The listing builds one solid part. Answer for the finished solid, in the listing's coordinates (mm). Coordinates: 2 decimals unless noted, no trailing zeros. Order: outer loops, then holes, each group sorted by start corner. A loop starts at its lowest first (then second) coordinate and runs counter-clockwise, first axis right, second up. Notation, with made-up numbers: (81.25, 82) - (109.25, 82) arc R27 ccw to (109.25, 100) - close; hole circle Ø6 at (10.25, 74.5). An arc over 180 degrees is marked (long way). Use one line per item in the form item = value. Start each with the question number.
Item 1: Section A-A, the plane z = 0 is taken. Write down the section's boundary in (x, y).
Item 2: The mould has two halves that part along Z. Classify faces 1 (the flat face through (0, 2, 25)), 2 (the flat face through (0, 0, 0)), 3 (the cylindrical face through (3.583, 2.169, -0.759)), 4 (the cylindrical face through (-10.417, 2.169, -0.759)): released by +Z, released by -Z, zero draft, split by the parting line, or undercut.
Item 3: Consider line 1 along X through (y, z) = (2.3, 0); line 2 along X through (y, z) = (3.45, -3); line 3 along Z through (x, y) = (8, 3.4). Determine where each line is inside the solid, lowest interval first. Write a range as [from, to].
Item 4: Each of these flat-tipped pins is pushed along its axis until it touches: pin 1 Ø2 at (y, z) = (0.5, 16.5) entering from +X; pin 2 Ø12 at (x, z) = (16.5, -4) entering from -Y. Where does it stop, or does it pass through?
Item 5: Section B-B, the plane x = 7 is taken. Write down the section's boundary in (y, z).
Item 6: Section D-D, the plane x = 14 is taken. Write down the section's boundary in (y, z), and give its area (3 significant figures).
Item 7: Section C-C, the plane y = 1 is taken. Write down the section's boundary in (x, z), and give its area (3 significant figures).
from build123d import *

# Parameters (mm, degrees)
SKETCH1_R           = 3.5
BOSS_EXTRUDE1_DEPTH = 4.4


with BuildPart() as part:
    # Sketch1 → Boss-Extrude1 (new body)
    with BuildSketch(Plane(origin=(0, 0, 0), x_dir=(1, 0, 0), z_dir=(0, 1, 0))):
        with BuildLine():
            Line((-23, 15), (23, 15))
            Line((23, 15), (23, -3))
            ThreePointArc((23, -3), (14.514718626, -6.514718626), (11, -15))
            ThreePointArc((11, -15), (12.426471853, -20.674548662), (16.366750419, -25))
            Line((16.366750419, -25), (-16.366750419, -25))
            ThreePointArc((-16.366750419, -25), (-12.426471853, -20.674548662), (-11, -15))
            ThreePointArc((-11, -15), (-14.514718626, -6.514718626), (-23, -3))
            Line((-23, -3), (-23, 15))
        make_face()
        with Locations(Location((-7, 0, 0), (0, 0, 270))):
            Circle(SKETCH1_R, mode=Mode.SUBTRACT)
        with Locations(Location((7, 0, 0), (0, 0, 270))):
            Circle(SKETCH1_R, mode=Mode.SUBTRACT)
    extrude(amount=BOSS_EXTRUDE1_DEPTH)


solid = part.part
Response:
q1.outline = (-23, 0) - (-10.5, 0) - (-10.5, 4.4) - (-23, 4.4) - close; (-3.5, 0) - (3.5, 0) - (3.5, 4.4) - (-3.5, 4.4) - close; (10.5, 0) - (23, 0) - (23, 4.4) - (10.5, 4.4) - close
q2.face_1 = released by +Z
q2.face_2 = zero draft
q2.face_3 = undercut
q2.face_4 = undercut
q3.line_1 = [-23, -10.5], [-3.5, 3.5], [10.5, 23]
q3.line_2 = [-23, -8.8], [-5.2, 5.2], [8.8, 23]
q3.line_3 = [-15, -3.35], [3.35, 25]
q4.pin_1 = 11.26
q4.pin_2 = 0
q5.outline = (0, -15) - (4.4, -15) - (4.4, -3.5) - (0, -3.5) - close; (0, 3.5) - (4.4, 3.5) - (4.4, 25) - (0, 25) - close
q6.outline = (0, -15) - (4.4, -15) - (4.4, 7.06) - (0, 7.06) - close; (0, 22.94) - (4.4, 22.94) - (4.4, 25) - (0, 25) - close
q6.area = 106 mm2
q7.outline = (-23, -15) - (23, -15) - (23, 3) arc R12 cw to (16.37, 25) - (-16.37, 25) arc R12 cw to (-23, 3) - close; hole circle Ø7 at (-7, 0); hole circle Ø7 at (7, 0)
q7.area = 1,330 mm2
